Study the drawing (mm; zero at the part's minimum x, y, z) and answer. Give positions to 0.01 mm unless a question says otherwise; leave off trailing zeros. Order: outer loops, then holes, each group sorted by start corner. A loop starts at its lowest first (then second) coordinate and runs counter-clockwise, first axis right, second up. Notation, with made-up numbers: (-27, 81) - (-1, 81) arc R31 cw to (-1, 117) - close; hole circle Ø1 at (1.5, 20.25). An arc over 180 degrees is marked (long way). Write each question's results on one line, items separated by ' | '. Start each with the question number.
1. Section D-D (z = 45.5) is taken. Give the vertices of the cut face in (x, y) (1 decimal), and give its area (3 significant figures).
2. Flat-ended cylindrical pins translate along their axes: pin 1 (5 mm diameter, centred on y = 8, z = 125.5, fed in from -X); pin 2 (1.5 mm diameter, centred on x = 231, y = 4.5, fed in from +Z); pin 3 (10 mm diameter, centred on x = 287.5, z = 200.5, fed in from +Y); pin 4 (2 mm diameter, centred on y = 7.5, z = 141.5, fed in from -X). Find the tip coordinate at first contact, or state that the pin passes through.
3. Section A-A (z = 200) is taken. Give the vertices of the cut face in (x, y).
4. Section C-C (x = 335) is taken. Give the vertices of the cut face in (y, z).
5. Section B-B (x = 247) is taken. Give the vertices of the cut face in (y, z).
6. Find the intervals of material crossed by L1, parallel to X at y = 4.75, z = 115 (1 decimal); L2, parallel to Z at x = 65, y = 6 (1 decimal); L3, parallel to X at y = 1.75, z = 165.5 (1 decimal), in increasing order.
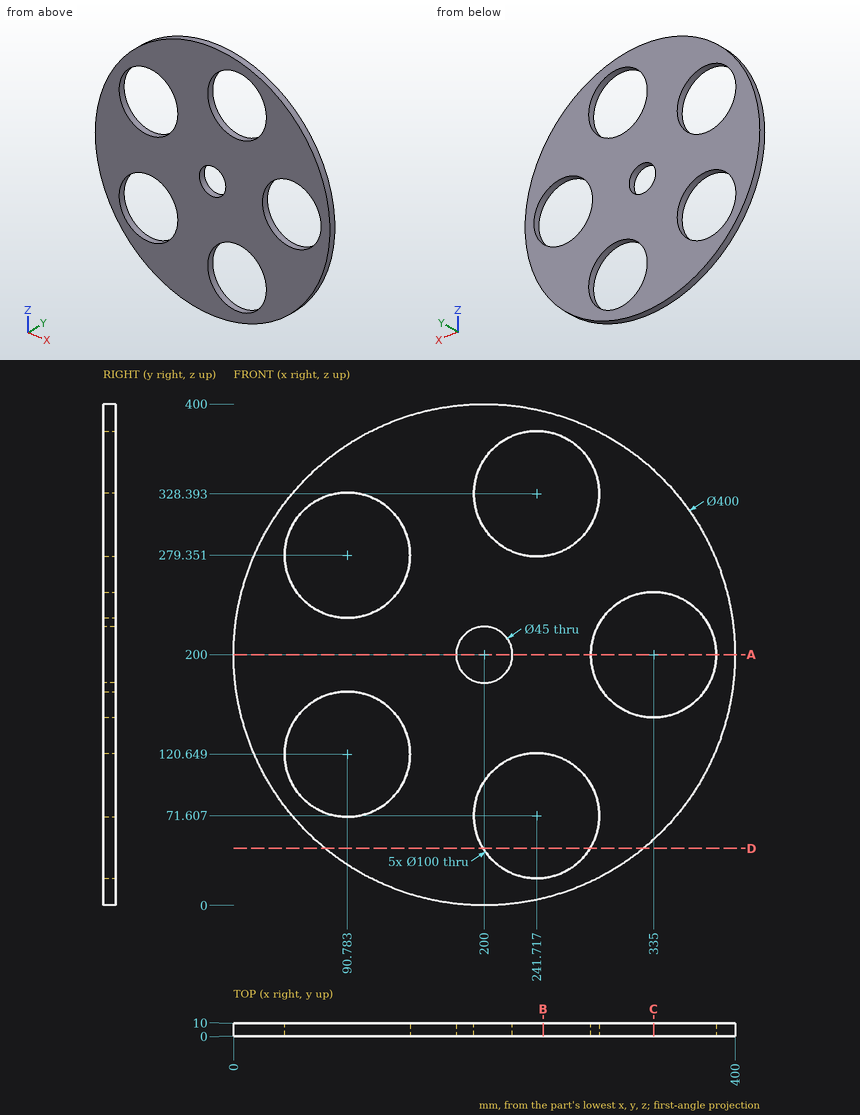
Reported:
1) outline: (73, 0) - (199.1, 0) - (199.1, 10) - (73, 10) - close; (284.4, 0) - (327, 0) - (327, 10) - (284.4, 10) - close | area: 1,690 mm²
2) pin 1: x = 13.41 | pin 2: z = 397.7 | pin 3: y = 10 | pin 4: x = 8.44
3) outline: (0, 0) - (177.5, 0) - (177.5, 10) - (0, 10) - close; (222.5, 0) - (285, 0) - (285, 10) - (222.5, 10) - close; (385, 0) - (400, 0) - (400, 10) - (385, 10) - close
4) outline: (0, 52.44) - (10, 52.44) - (10, 150) - (0, 150) - close; (0, 250) - (10, 250) - (10, 347.56) - (0, 347.56) - close
5) outline: (0, 5.6) - (10, 5.6) - (10, 21.89) - (0, 21.89) - close; (0, 121.33) - (10, 121.33) - (10, 278.67) - (0, 278.67) - close; (0, 378.11) - (10, 378.11) - (10, 394.4) - (0, 394.4) - close
6) L1: 19 to 41.1, 140.5 to 216.9, 266.6 to 381 | L2: 52.4 to 77.8, 163.5 to 236.5, 322.2 to 347.6 | L3: 3 to 68.7, 112.9 to 298.8, 371.2 to 397
